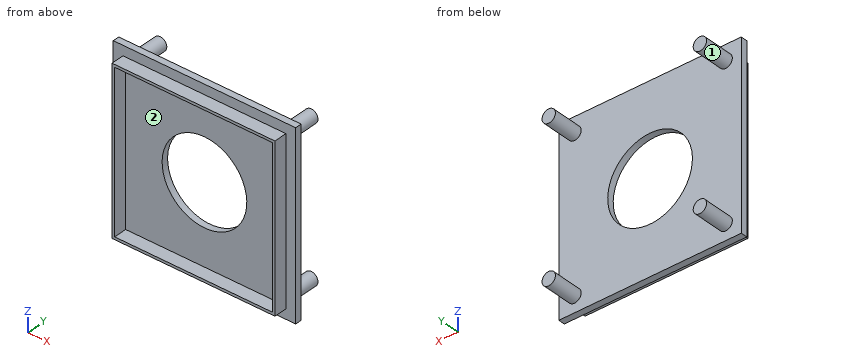
```python
from build123d import *

# Parameters (mm, degrees)
SKETCH1_W           = 140
SKETCH1_H           = 140
BOSS_EXTRUDE1_DEPTH = 5
CUT_EXTRUDE1_REACH  = 101.121
SKETCH3_R           = 32.5
SKETCH4_R           = 5.125
BOSS_EXTRUDE2_DEPTH = 23.5
SKETCH5_W           = 125
SKETCH5_H           = 125
SKETCH5_W_2         = 121
SKETCH5_H_2         = 121
BOSS_EXTRUDE3_DEPTH = 10


with BuildPart() as part:
    # Sketch1 → Boss-Extrude1 (new body)
    with BuildSketch(Plane(origin=(0, 0, 0), x_dir=(1, 0, 0), z_dir=(0, 1, 0))):
        Rectangle(SKETCH1_W, SKETCH1_H)
    extrude(amount=BOSS_EXTRUDE1_DEPTH)

    # Sketch3 → Cut-Extrude1 (cut, up to next)
    with BuildSketch(Plane(origin=(0, 5, 0), x_dir=(1, 0, 0), z_dir=(0, 1, 0)), mode=Mode.PRIVATE) as cut_extrude1_sk1:
        with Locations(Location((0, 0, 0), (0, 0, 270))):
            Circle(SKETCH3_R)
    cut_extrude1_tool1 = extrude(cut_extrude1_sk1.sketch, amount=-CUT_EXTRUDE1_REACH, mode=Mode.PRIVATE) & part.part
    add(cut_extrude1_tool1.solids().sort_by_distance((0, 5, 0))[0], mode=Mode.SUBTRACT)

    # Sketch4 → Boss-Extrude2 (add)
    with BuildSketch(Plane(origin=(0, 5, 0), x_dir=(1, 0, 0), z_dir=(0, 1, 0))):
        with Locations(Location((-58, 58, 0), (0, 0, 90))):
            Circle(SKETCH4_R)
        with Locations(Location((58, 58, 0), (0, 0, 90))):
            Circle(SKETCH4_R)
        with Locations(Location((58, -58, 0), (0, 0, 90))):
            Circle(SKETCH4_R)
        with Locations(Location((-58, -58, 0), (0, 0, 90))):
            Circle(SKETCH4_R)
    extrude(amount=BOSS_EXTRUDE2_DEPTH)

    # Sketch5 → Boss-Extrude3 (add)
    with BuildSketch(Plane.XZ):
        Rectangle(SKETCH5_W, SKETCH5_H)
        Rectangle(SKETCH5_W_2, SKETCH5_H_2, mode=Mode.SUBTRACT)
    extrude(amount=BOSS_EXTRUDE3_DEPTH)


solid = part.part
```
The listing builds one solid part. Answer for the finished solid, in the listing's coordinates (mm). Face numbers are marked on the shaded views. A direction names the side the tool comes from. Coordinates: 2 decimals unless noted, no trailing zeros. Write each loop counter-clockwise with the first axis right and the second up, starting at its lowest first coordinate (ties: lowest second). Pieces come first, ordered by that corner, then holes. Notation, with made-up numbers: (-35.5, -31) - (22.5, -31) arc R8 cw to (22.5, -26) - close; hole circle Ø6 at (55, -8). An arc over 180 degrees is marked (long way). Return JSON: item names as keys, results as strings. Group by question number.
1. A cutting plane is placed at C-C, the plane z = 58. Determine the outline of the cut face in (x, y) (3 decimals).
2. A cutting plane is placed at A-A, the plane z = 0. Determine the outline of the cut face in (x, y).
3. A cutting plane is placed at D-D, the plane y = 24. Determine the outline of the cut face in (x, z) (3 decimals), plus the area to 3 significant figures.
4. Which of the six approach directions +Z, -Z, +X, -X, +Y, -Y give full straight-line access (tool end or side, diameter ignored) to the marked faces 1 and 2?
5. Given pin 1 (3 mm diameter, centred on x = -48.5, z = 43.5, fed in from -Y); pin 2 (4 mm diameter, centred on x = -26, z = -33, fed in from +Y); pin 3 (11 mm diameter, centred on y = -6, z = -16.5, fed in from -X), each flat-ended and moving along its own axis, determine where each tip first touches the part or whether it passes through.
6. A cutting plane is placed at B-B, the plane x = 0. Determine the outline of the cut face in (y, z).
7. Straight lines are drawn through the part: L1, parallel to Z at x = -31.5, y = -6; L2, parallel to X at y = 1, z = 0; L3, parallel to Y at x = -29, z = -56. For each, find the intervals that lie inside material, in ascending order.
Ans:
{
 "1": {"outline": "(-70, 0) - (-62.5, 0) - (-62.5, -10) - (-60.5, -10) - (-60.5, 0) - (60.5, 0) - (60.5, -10) - (62.5, -10) - (62.5, 0) - (70, 0) - (70, 5) - (63.125, 5) - (63.125, 28.5) - (52.875, 28.5) - (52.875, 5) - (-52.875, 5) - (-52.875, 28.5) - (-63.125, 28.5) - (-63.125, 5) - (-70, 5) - close"},
 "2": {"outline": "(-70, 0) - (-62.5, 0) - (-62.5, -10) - (-60.5, -10) - (-60.5, 0) - (-32.5, 0) - (-32.5, 5) - (-70, 5) - close; (32.5, 0) - (60.5, 0) - (60.5, -10) - (62.5, -10) - (62.5, 0) - (70, 0) - (70, 5) - (32.5, 5) - close"},
 "3": {"outline": "circle Ø10.25 at (-58, -58); circle Ø10.25 at (-58, 58); circle Ø10.25 at (58, -58); circle Ø10.25 at (58, 58)", "area": "330 mm²"},
 "4": {"face 1": "+Y", "face 2": "-Y"},
 "5": {"pin 1": "y = 0", "pin 2": "y = 5", "pin 3": "x = -62.5"},
 "6": {"outline": "(-10, -62.5) - (0, -62.5) - (0, -70) - (5, -70) - (5, -32.5) - (0, -32.5) - (0, -60.5) - (-10, -60.5) - close; (-10, 60.5) - (0, 60.5) - (0, 32.5) - (5, 32.5) - (5, 70) - (0, 70) - (0, 62.5) - (-10, 62.5) - close"},
 "7": {"L1": "-62.5 to -60.5, 60.5 to 62.5", "L2": "-70 to -32.5, 32.5 to 70", "L3": "0 to 5"}
}
